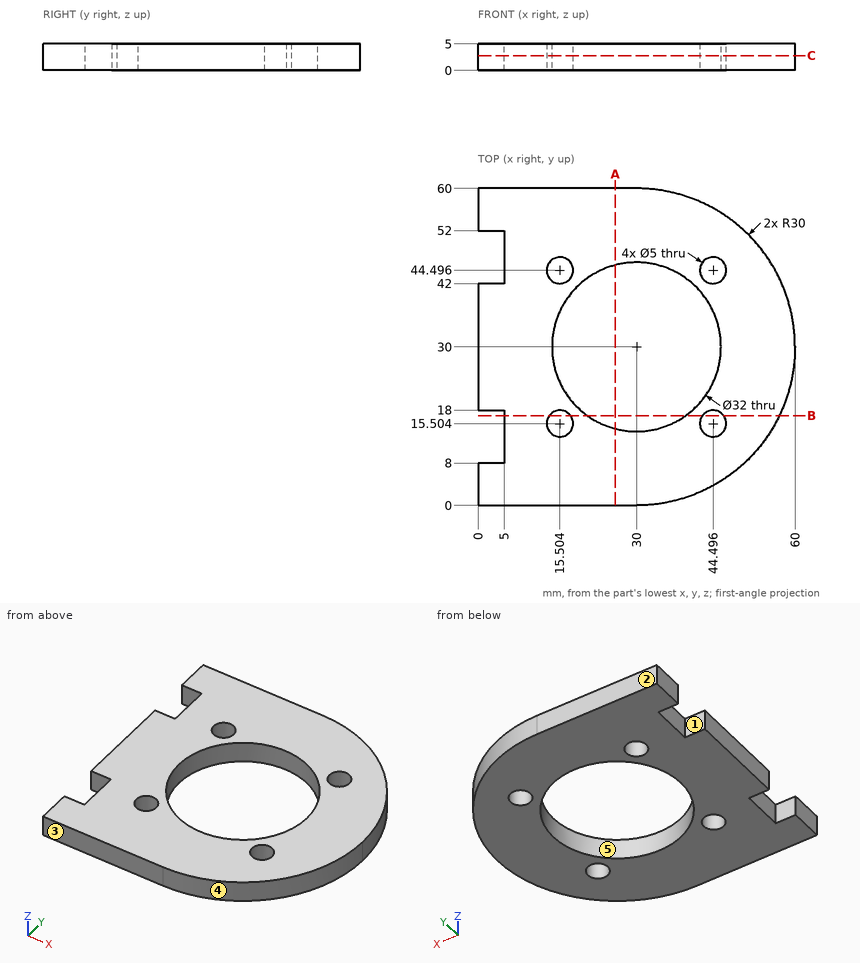
Geometry: see drawing. Coordinates: mm, zero at the bounding-box minimum. A direction names the side the tool comes from. Round coordinates to 2 decimals unless told otherwise and drop trailing zeros. Write each loop counter-clockwise with the first axis right and the second up, starting at its lowest first coordinate (ties: lowest second). Pieces come first, ordered by that corner, then holes.
1) Cut plane B-B (y = 17). Return the cut outline in (x, z).
2) Ray query, L1, parallel to Y at x = 29.5, z = 0.9; L2, parallel to X at y = 16.5, z = 3.05 (1 decimal); L3, parallel to X at y = 16, z = 3.65 (1 decimal). Return the intervals inside material, ascending.
3) Draft query along X for the marked faces 3, 4 and 5. Return one class per face: pulls with the +X half, pulls with the -X half, needs draft (parallel to the pull), parting line crosses it, or undercut.
4) Cut plane C-C (z = 2.8). Count the separate pieces of the cut face and the enclosed holes in it, then the cut area to 3 significant figures.
5) Cut plane A-A (x = 26). Return the cut outline in (y, z), then the cut area to 3 significant figures.
6) Reachability of the marked faces 1 and 2 from +Z, -Z, +X, -X, +Y, -Y: full face, straight path, thin tool, end or side. Return the list, or none.
7) Contact query for flat-ended pins moving along their axis: P1, Ø2.5, axis at y = 47, z = 2, coming from the -X side; P2, Ø1, axis at y = 25, z = 4, coming from the +X side. Output: stop coordinate, or through.
Geometry says:
1. outline: (5, 0) - (13.5, 0) - (13.5, 5) - (5, 5) - close; (17.51, 0) - (20.67, 0) - (20.67, 5) - (17.51, 5) - close; (39.33, 0) - (42.49, 0) - (42.49, 5) - (39.33, 5) - close; (46.5, 0) - (57.04, 0) - (57.04, 5) - (46.5, 5) - close
2. L1: y = 0 to 14.01, 45.99 to 60
2. L2: x = 5 to 13.2, 17.8 to 21.4, 38.6 to 42.2, 46.8 to 56.8
2. L3: x = 5 to 13.1, 18 to 22.3, 37.7 to 42, 46.9 to 56.5
3. face 3: needs draft
3. face 4: pulls with the +X half
3. face 5: undercut
4. separate pieces: 1
4. enclosed holes: 5
4. area: 2,230 mm2
5. outline: (0, 0) - (14.51, 0) - (14.51, 5) - (0, 5) - close; (45.49, 0) - (60, 0) - (60, 5) - (45.49, 5) - close
5. area: 145 mm2
6. face 1: +Z, -Z, -X
6. face 2: +Z, -Z, +X, -X, +Y
7. P1: stops at x = 5
7. P2: stops at x = 59.66
